```python
from build123d import *

# Parameters (mm, degrees)
AUFSATZ_LINEAR_AUSTRAGEN1_DEPTH = 90
F_5_0_5_DURCHMESSER_BOHRUNG1_D  = 5
F_5_0_5_DURCHMESSER_BOHRUNG2_D  = 5


with BuildPart() as part:
    # Skizze2 → Aufsatz-Linear austragen1 (new body)
    with BuildSketch(Plane.XY):
        with BuildLine():
            ThreePointArc((6, 13), (8.050252532, 8.050252532), (13, 6))
            Line((13, 6), (60.7, 6))
            ThreePointArc((60.7, 6), (62.326345597, 5.326345597), (63, 3.7))
            Line((63, 3.7), (63, 0))
            Line((63, 0), (0, 0))
            Line((0, 0), (0, 63))
            Line((0, 63), (3.7, 63))
            ThreePointArc((3.7, 63), (5.326345597, 62.326345597), (6, 60.7))
            Line((6, 60.7), (6, 13))
        make_face()
    extrude(amount=AUFSATZ_LINEAR_AUSTRAGEN1_DEPTH)

    # Ø5.0 (5) Durchmesser Bohrung1 (through all)
    with Locations(Plane(origin=(6, 25, 67.5), x_dir=(0, 1, 0), z_dir=(1, 0, 0))):
        with Locations((0, 0), (24, 0), (24, -22.5), (0, -22.5), (0, -45), (24, -45)):
            Hole(F_5_0_5_DURCHMESSER_BOHRUNG1_D / 2)

    # Ø5.0 (5) Durchmesser Bohrung2 (through all)
    with Locations(Plane(origin=(49, 6, 67.5), x_dir=(0, 0, 1), z_dir=(0, 1, 0))):
        with Locations((0, 0), (-22.5, 0), (-22.5, -24), (0, -24), (-59.5, -24), (-59.5, -9), (-59.5, 7)):
            Hole(F_5_0_5_DURCHMESSER_BOHRUNG2_D / 2)


solid = part.part
```
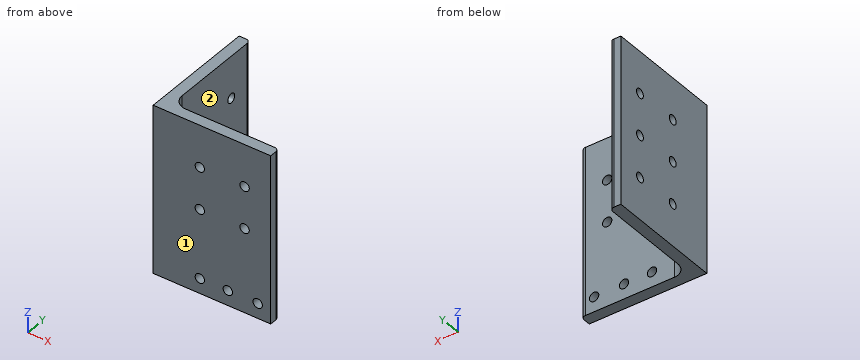
For this review, take the finished solid that the model builds, in its own axes (mm). Face numbers are marked on the shaded views. A direction names the side the tool comes from. Give positions to 0.01 mm unless a question says otherwise; leave off trailing zeros. Write each loop counter-clockwise with the first axis right and the second up, starting at its lowest first coordinate (ties: lowest second). Pieces come first, ordered by that corner, then holes. Notation, with made-up numbers: M 51.25,-16 L 65.25,-16 A22 cw 65.25,1 Z; hole C -35,52 d1. An arc over 180 degrees is marked long. Answer as a JSON object with one key per item and string values. Group by question number.
Item 1: Consider section B-B on z = 67.5. Write out the cut boundary in (x, y).
Item 2: Tool access review of the marked faces 1 and 2: name each direction out of +Z, -Z, +X, -X, +Y, -Y from which nothing blocks a thin tool from reaching the whole face with its end or side.
Item 3: Consider section D-D on y = 25. Write out the cut boundary in (x, z).
Item 4: For probe 1 along Z at (x, y) = (2, 25); probe 2 along X at (y, z) = (19.5, 53), list the stretches that pass through material, from the lowest coordinate up. Write a range as [from, to].
Item 5: Consider section C-C on x = 49. Write out the cut boundary in (y, z), plus the area to 3 significant figures.
Item 6: For pin 1 Ø4.5 at (y, z) = (25, 67.5) entering from +X; pin 2 Ø6 at (x, z) = (49, 45) entering from +Y; pin 3 Ø24 at (y, z) = (33, 36) entering from +X, all flat-tipped, find the tip position at first contact; note any pin that passes through.
Item 7: Consider section A-A on x = 25. Write out the cut boundary in (y, z), plus the area to 3 significant figures.
Check result:
{
 "1": {"outline": "M 0,0 L 22.5,0 L 22.5,6 L 13,6 A7 cw 6,13 L 6,22.5 L 0,22.5 Z; M 0,27.5 L 6,27.5 L 6,46.5 L 0,46.5 Z; M 0,51.5 L 6,51.5 L 6,60.7 A2.3 ccw 3.7,63 L 0,63 Z; M 27.5,0 L 46.5,0 L 46.5,6 L 27.5,6 Z; M 51.5,0 L 63,0 L 63,3.7 A2.3 ccw 60.7,6 L 51.5,6 Z"},
 "2": {"face 1": "+Z, -Z, +X, -X, -Y", "face 2": "+Z, -Z, +X, +Y"},
 "3": {"outline": "M 0,0 L 6,0 L 6,20 L 0,20 Z; M 0,25 L 6,25 L 6,42.5 L 0,42.5 Z; M 0,47.5 L 6,47.5 L 6,65 L 0,65 Z; M 0,70 L 6,70 L 6,90 L 0,90 Z"},
 "4": {"probe 1": "z = [0, 20], [25, 42.5], [47.5, 65], [70, 90]", "probe 2": "x = [0, 6]"},
 "5": {"outline": "M 0,0 L 6,0 L 6,42.5 L 0,42.5 Z; M 0,47.5 L 6,47.5 L 6,65 L 0,65 Z; M 0,70 L 6,70 L 6,90 L 0,90 Z", "area": "480 mm^2"},
 "6": {"pin 1": "passes through", "pin 2": "stops at y = 6", "pin 3": "stops at x = 6"},
 "7": {"outline": "M 0,0 L 6,0 L 6,5.5 L 0,5.5 Z; M 0,10.5 L 6,10.5 L 6,42.5 L 0,42.5 Z; M 0,47.5 L 6,47.5 L 6,65 L 0,65 Z; M 0,70 L 6,70 L 6,90 L 0,90 Z", "area": "450 mm^2"}
}
